Autodesk Inventor part; units mm, degrees
ref_plane "YZ Plane" through (0, 0, 0) normal (1, 0, 0) x (0, 1, 0)
ref_plane "XZ Plane" through (0, 0, 0) normal (0, 1, 0) x (-1, 0, 0)
ref_plane "XY Plane" through (0, 0, 0) normal (0, 0, 1) x (1, 0, 0)
sketch "スケッチ1" plane through (0, 0, 0) normal (0, 1, 0) x (-1, 0, 0)
  line L0 (5, -10) -> (-5, -10)
  line L1 (-5, -10) -> (-5, 10)
  line L2 (-5, 10) -> (5, 10)
  line L3 (5, 10) -> (5, -10)
  line L4 (5, -10) -> (-5, 10) construction
  line L5 (-5, -10) -> (5, 10) construction
  point P0 (0, 0)
  dimension "d0" = 10
  dimension "d1" = 20
extrude "押し出し1" add sketch "スケッチ1" along normal blind 6
sketch "スケッチ2" plane through (0, 0, 0) normal (0, -1, 0) x (1, 0, 0)
  line L0 (5, 10) -> (5, -10)
  circle A0 centre (5, 0) radius 6.75
  point P0 (0, 0)
  point P1 (5, -6.75)
  point P2 (5, 6.75)
  dimension "d4" = 13.5
extrude "押し出し2" cut sketch "スケッチ2" against normal blind 3 contours L0 A0 picked at (3.1483, 1.2781)
sketch "スケッチ3" plane through (0, 0, 0) normal (0, -1, 0) x (1, 0, 0)
  line L0 (-5, 10) -> (5, 10)
  line L1 (5, 10) -> (5, -10)
  line L2 (5, -10) -> (-5, -10)
  line L3 (-5, -10) -> (-5, 10)
  line L4 (-5, 10) -> (5, -10) construction
  line L5 (5, 10) -> (-5, -10) construction
  point P0 (0, 0)
  dimension "d7" = 10
  dimension "d8" = 20
extrude "押し出し3" add sketch "スケッチ3" along normal blind 2
sketch "スケッチ4" plane through (0, 6, 0) normal (0, 1, 0) x (1, 0, 0)
  line L0 (5, 7) -> (0, 7)
  line L1 (0, 7) -> (0, -7)
  line L2 (0, -7) -> (5, -7)
  line L3 (5, -7) -> (5, 7)
  line L4 (5, -10) -> (5, 10)
  point P0 (0, 0)
  dimension "d11" = 5
  dimension "d12" = 14
  dimension "d13" = 5
  dimension "d14" = 7
extrude "押し出し4" add sketch "スケッチ4" along normal blind 120
fillet "フィレット1" radius 2 3 edges at (2.5, 6, 7) (2.5, 6, -7) (0, 6, 0)
fillet "フィレット2" radius 0.2 12 edges at (-0.5858, 6.5858, -7.5858) (0, 67, -7) (-0.5858, 6.5858, 7.5858) (0, 67, 7) (2.5, 126, 7) (0, 126, 0) (2.5, 126, -7) (0, 6, -10) (-5, 6, 0) (0, 6, 10) (-5, 2, 10) (-5, 2, -10)
sketch "スケッチ5" plane through (0, 8, 6.8) normal (-1, 0, 0) x (0, 0, 1)
  line L0 (3, -2) -> (-16.6, -2)
  line L1 (-13.8, 117.8) -> (-13.8, 0)
  point P0 (-6.8, -8)
  point P1 (-6.8, 28)
  point P2 (-6.8, 108)
  dimension "d19" = 30
  dimension "d20" = 80
  dimension "d21" = 7
  dimension "d22" = 7
hole "穴1" at (0, 36, 0) at (0, 116, 0) direction (1, 0, 0) diameter 6 end through all
properties part number "baseB"
Can you work these out from the model? Positions are in its coordinate system, mm. A direction names the side the tool comes from. Give positions to 0.01 mm unless a question says otherwise; leave off trailing zeros. Order: outer loops, then holes, each group sorted by start corner. A loop starts at its lowest first (then second) coordinate and runs counter-clockwise, first axis right, second up. Notation, with made-up numbers: (31, 57) - (85, 57) arc R16 cw to (85, 65) - close; hole circle Ø3 at (73, 70.5). An arc over 180 degrees is marked (long way). Write each question's results on one line, items separated by ' | '.
1) If we mould it in two halves opening along Z, with no side actions, what happens to faces 6 (the face through (-1.75, 1.48, 0.15)), 7 (the face through (3, 66, 7)), 8 (the face through (3, 126, 0))? For each: pulls with the +Z half, pulls with the -Z half, needs draft (parallel to the pull), parting line crosses it, or undercut.
Final values:
face 6: undercut | face 7: pulls with the +Z half | face 8: needs draft
2) I'm going to push flat-ended pins straight in: pin 1 Ø4 at (y, z) = (37, -1) entering from -X; pin 2 Ø2.5 at (x, y) = (2.5, 52.5) entering from +Z; pin 3 Ø4 at (x, y) = (3.5, 83) entering from -Z. Where does each tip first touch, or does it pass through?
Final values:
pin 1: stops at x = 0 | pin 2: stops at z = 7 | pin 3: stops at z = -7
3) On a 3-axis mill with a long thin cutter (end or side, diameter ignored), from which of +Z, -Z, +X, -X, +Y, -Y can I reach the whole of each face in a straight line? I mean faces 1 (the face through (2.33, 6.57, 7.6)), 2 (the face through (2, 3, 0)), 3 (the face through (3, 66, -7)), 4 (the face through (3, 113, 0)), 5 (the face through (0, 66, 0)). Say none if no direction works.
Final values:
face 1: +Z, +X, -X, +Y | face 2: +X | face 3: -Z, +X, -X, +Y | face 4: +X, -X | face 5: +Z, -Z, -X, +Y
4) Suppose I cut it at A-A, the plane y = 36. Write out the boundary of the cut face in (x, z).
Final values:
outline: (0, -6.8) arc R0.2 ccw to (0.2, -7) - (5, -7) - (5, -3) - (0, -3) - close; (0, 3) - (5, 3) - (5, 7) - (0.2, 7) arc R0.2 ccw to (0, 6.8) - close
5) Please list where these lines run through material, in increasing order: line 1 along Y through (x, z) = (3.3, 0); line 2 along Y through (x, z) = (1.5, -5.25); line 3 along Z through (x, y) = (1.9, 36). Write a range as [from, to].
Final values:
line 1: y = [-2, 0], [3, 33], [39, 113], [119, 126] | line 2: y = [-2, 0], [3, 126] | line 3: z = [-7, -3], [3, 7]
6) Suppose I cut it at C-C, the plane x = 3.75. Write out the boundary of the cut face in (y, z), then the cut area to 3 significant figures.
Final values:
outline: (-2, -10) - (5.8, -10) arc R0.2 ccw to (6, -9.8) - (6, -9) arc R2 cw to (8, -7) - (125.8, -7) arc R0.2 ccw to (126, -6.8) - (126, 6.8) arc R0.2 ccw to (125.8, 7) - (8, 7) arc R2 cw to (6, 9) - (6, 9.8) arc R0.2 ccw to (5.8, 10) - (-2, 10) - close; hole (0, -6.63) - (3, -6.63) - (3, 6.63) - (0, 6.63) - close; hole circle Ø6 at (36, 0); hole circle Ø6 at (116, 0) | area: 1,750 mm^2
7) Suppose I cut it at B-B, the plane z = 0. Write out the boundary of the cut face in (x, y), then the cut area to 3 significant figures.
Final values:
outline: (-5, -2) - (5, -2) - (5, 0) - (-1.75, 0) - (-1.75, 3) - (5, 3) - (5, 33) - (0, 33) - (0, 8) arc R2 cw to (-2, 6) - (-4.8, 6) arc R0.2 ccw to (-5, 5.8) - close; (0, 39) - (5, 39) - (5, 113) - (0, 113) - close; (0, 119) - (5, 119) - (5, 126) - (0.2, 126) arc R0.2 ccw to (0, 125.8) - close | area: 601 mm^2
